from build123d import *

# Parameters (mm, degrees)
BOSS_EXTRUDE1_DEPTH                                 = 46.355
SKETCH3_W                                           = 86.36
SKETCH3_H                                           = 3.683
BOSS_EXTRUDE2_DEPTH                                 = 11.176
SKETCH3_3_W                                         = 86.36
SKETCH3_3_H                                         = 9.271
BOSS_EXTRUDE3_DEPTH                                 = 5.588
SKETCH4_W                                           = 22.86
SKETCH4_H                                           = 3.81
BOSS_EXTRUDE4_DEPTH                                 = 5.588
CBORE_FOR_10_BINDING_HEAD_MACHINE_SCREW_D           = 5.1054
CBORE_FOR_10_BINDING_HEAD_MACHINE_SCREW_CBORE_D     = 11.1125
CBORE_FOR_10_BINDING_HEAD_MACHINE_SCREW_CBORE_DEPTH = 7.747


with BuildPart() as part:
    # Sketch2 → Boss-Extrude1 (new body, symmetric)
    with BuildSketch(Plane(origin=(0, 0, 0), x_dir=(0, 0, -1), z_dir=(1, 0, 0))):
        Polygon((19.05, 0), (19.05, -11.176), (57.15, -11.176), (57.15, -4.826), (25.4, 6.35), (0, 6.35), (0, 0), align=None)
    extrude(amount=BOSS_EXTRUDE1_DEPTH, both=True)

    # Sketch3 → Boss-Extrude2 (add)
    with BuildSketch(Plane.XZ):
        with Locations((0, -17.2085)):
            Rectangle(SKETCH3_W, SKETCH3_H)
    extrude(amount=BOSS_EXTRUDE2_DEPTH)

    # Sketch3<3> → Boss-Extrude3 (add)
    with BuildSketch(Plane.XZ):
        with Locations((0, -10.7315)):
            Rectangle(SKETCH3_3_W, SKETCH3_3_H)
    extrude(amount=BOSS_EXTRUDE3_DEPTH)

    # Sketch4 → Boss-Extrude4 (add)
    with BuildSketch(Plane.XZ.offset(5.588)):
        with Locations((-29.21, -9.271)):
            Rectangle(SKETCH4_W, SKETCH4_H)
        with Locations((29.21, -9.271)):
            Rectangle(SKETCH4_W, SKETCH4_H)
    extrude(amount=BOSS_EXTRUDE4_DEPTH)

    # CBORE for #10 Binding Head Machine Screw1 (through all)
    with Locations(Plane(origin=(0, 6.35, 0), x_dir=(-1, 0, 0), z_dir=(0, 1, 0))):
        with Locations((-31.75, -41.275), (0, -41.275), (31.75, -41.275)):
            CounterBoreHole(CBORE_FOR_10_BINDING_HEAD_MACHINE_SCREW_D / 2, CBORE_FOR_10_BINDING_HEAD_MACHINE_SCREW_CBORE_D / 2, CBORE_FOR_10_BINDING_HEAD_MACHINE_SCREW_CBORE_DEPTH)


solid = part.part
Geometry check sheet. Reference: the model listing, model coordinates, mm. A direction names the side the tool comes from. Coordinates: 2 decimals unless noted, no trailing zeros. Order: outer loops, then holes, each group sorted by start corner. A loop starts at its lowest first (then second) coordinate and runs counter-clockwise, first axis right, second up. Notation, with made-up numbers: (84, -9.75) - (124, -9.75) arc R27 ccw to (124, 14.25) - close; hole circle Ø1 at (61, -22.75). An arc over 180 degrees is marked (long way). Answer in a Markdown table with one row per item. Add a question column.
1) Cross-section at C-C, the plane x = 0. Record the cut outline in (y, z), then the cut area to 3 significant figures.
2) Set-up check for faces 5 (the flat face through (43.18, -4, -14)), 6 (the flat face through (29, -1.397, -42)), 7 (the flat face through (-1, -8, -15.367)): record each of +Z, -Z, +X, -X, +Y, -Y from which the full face is reachable in a straight line by a thin tool's end or side.
3) Release check for a two-part mould opening along X. For faces 1 (the flat face through (-1, -1.397, -44)), 2 (the flat face through (-46.355, -2, -28)), 3 (the flat face through (1, -8, -57.15)), 4 (the flat face through (40.64, -8, -9)) record: +X half, -X half, draft (parallel to the pull), parting line (faces both ways), or undercut.
4) Cross-section at A-A, the plane y = -9.5. Record the cut outline in (x, z) (3 decimals).
5) Cross-section at D-D, the plane x = 10. Record the cut outline in (y, z).
6) Cross-section at B-B, the plane x = 39. Record the cut outline in (y, z).
7) Gauge pin test, flat ends, axial feed: P1, Ø1.9, axis at y = -7.5, z = -8.5, coming from the -X side; P2, Ø4.5, axis at x = 34, y = -9.5, coming from the +Z side; P3, Ø1.9, axis at y = -8, z = -9, coming from the +X side. Record the tip position at first contact, or that the pin passes through.
8) Material ranges on line 1 along X through (y, z) = (-6, -9); line 2 along Z through (x, y) = (0, -7); line 3 along Z through (x, y) = (-28.5, -9.5), recorded low to high. Write a range as [from, to].
Check result:
| question | item | result |
|---|---|---|
| 1 | outline | (-11.18, -57.15) - (-4.83, -57.15) - (-1.19, -46.83) - (-1.4, -46.83) - (-1.4, -43.83) - (-11.18, -43.83) - close; (-11.18, -38.72) - (-1.4, -38.72) - (-1.4, -35.72) - (2.72, -35.72) - (6.35, -25.4) - (6.35, 0) - (0, 0) - (0, -6.1) - (-5.59, -6.1) - (-5.59, -15.37) - (-11.18, -15.37) - close |
| 1 | area | 630 mm² |
| 2 | face 5 | +Z, +X, -Y |
| 2 | face 6 | +Y |
| 2 | face 7 | +X, -X, -Y |
| 3 | face 1 | undercut |
| 3 | face 2 | -X half |
| 3 | face 3 | draft |
| 3 | face 4 | +X half |
| 4 | outline | (-46.355, -57.15) - (46.355, -57.15) - (46.355, -19.05) - (43.18, -19.05) - (43.18, -15.367) - (-43.18, -15.367) - (-43.18, -19.05) - (-46.355, -19.05) - close; (-40.64, -11.176) - (-17.78, -11.176) - (-17.78, -7.366) - (-40.64, -7.366) - close; (17.78, -11.176) - (40.64, -11.176) - (40.64, -7.366) - (17.78, -7.366) - close; hole circle Ø5.105 at (-31.75, -41.275); hole circle Ø5.105 at (0, -41.275); hole circle Ø5.105 at (31.75, -41.275) |
| 5 | outline | (-11.18, -57.15) - (-4.83, -57.15) - (6.35, -25.4) - (6.35, 0) - (0, 0) - (0, -6.1) - (-5.59, -6.1) - (-5.59, -15.37) - (-11.18, -15.37) - close |
| 6 | outline | (-11.18, -57.15) - (-4.83, -57.15) - (6.35, -25.4) - (6.35, 0) - (0, 0) - (0, -6.1) - (-5.59, -6.1) - (-5.59, -7.37) - (-11.18, -7.37) - (-11.18, -11.18) - (-5.59, -11.18) - (-5.59, -15.37) - (-11.18, -15.37) - close |
| 7 | P1 | stops at x = -40.64 |
| 7 | P2 | stops at z = -7.37 |
| 7 | P3 | stops at x = 40.64 |
| 8 | line 1 | x = [-40.64, -17.78], [17.78, 40.64] |
| 8 | line 2 | z = [-57.15, -43.83], [-38.72, -15.37] |
| 8 | line 3 | z = [-57.15, -15.37], [-11.18, -7.37] |
